Solid Edge part; units mm, degrees
sketch "Sketch1" plane through (0, 0, 0) normal (0, 0, 1) x (1, 0, 0)
  circle A0 centre (0, 0) radius 3.5
extrude "Protrusion1" add sketch "Sketch1" along normal blind 4
sketch "Sketch2" plane through (0, 0, 0) normal (0, 0, -1) x (1, 0, 0)
  circle A0 centre (0, 0) radius 2
extrude "Protrusion2" add sketch "Sketch2" along normal blind 16
sketch "Sketch3" plane through (0, 0, -16) normal (0, 0, -1) x (1, 0, 0)
  circle A0 centre (0, 0) radius 1.9997
extrude "Cutout1" cut sketch "Sketch3" against normal blind 15.984 flip side to cut
chamfer "Chamfer_1" distance 0.3 angle 45 1 edges at (-1.9997, 0, -16)
sketch "Sketch4" plane through (0, 0, 4) normal (0, 0, 1) x (1, 0, 0)
  line L0 (-0.866, 1.5) -> (0.866, 1.5)
  line L1 (1.7321, 0) -> (0.866, 1.5)
  line L2 (0.866, -1.5) -> (1.7321, 0)
  line L3 (-0.866, -1.5) -> (0.866, -1.5)
  line L4 (-1.7321, 0) -> (-0.866, -1.5)
  line L5 (-0.866, 1.5) -> (-1.7321, 0)
extrude "Cutout2" cut sketch "Sketch4" against normal blind 2
properties part number "24104709" material "Steel"
Build history of the part. All positions in model axes, mm. A direction names the side the tool comes from. Round coordinates to 2 decimals unless told otherwise and drop trailing zeros. Loops run counter-clockwise (first coordinate to the right, second up) from the corner with the lowest first, then second, coordinate; pieces in that order, holes last.
Item 1: Saw through at C-C (y = -2.25). List the corners of the cut face in (x, z).
Item 2: Which spindle directions (+Z, -Z, +X, -X, +Y, -Y) get a long thin tool onto all of the face, cutting with end or side? Do faces 1 (the face through (2, -2, 0)), 2 (the face through (0, 0, 2)), 3 (the face through (3.233, 1.341, 1.972)). Say none if no direction does.
Item 3: Saw through at B-B (z = -9). List the corners of the cut face in (x, y).
Item 4: Drill centre lines: line 1 along Y through (x, z) = (1, -14.75); line 2 along Y through (x, z) = (-0.75, 3.25). Where is each one in solid material? Low to high.
Item 5: Pin check, flat tip, straight feed: P1, Ø4, axis at x = 2, z = -12.5, coming from the -Y side. Stop position of the tip, or through.
Item 6: Two-plate mould, pull along Y, no slides. Class faces 4 (the face through (0, -2, 4)), 5 (the face through (0.923, 1.774, -7.968)), 6 (the face through (1.305, 0.74, 3.014)), 7 (the face through (0, 1.5, 3)): released by +Y, released by -Y, zero draft, split by the parting line, or undercut.
Worked answers:
1. outline: (-2.68, 0) - (2.68, 0) - (2.68, 4) - (-2.68, 4) - close
2. face 1: -Z
2. face 2: +Z
2. face 3: +Z, -Z
3. outline: circle Ø4 at (0, 0)
4. line 1: y = -1.73 to 1.73
4. line 2: y = -3.42 to -1.5, 1.5 to 3.42
5. P1: stops at y = -2
6. face 4: zero draft
6. face 5: split by the parting line
6. face 6: undercut
6. face 7: undercut
